Geometry check sheet. Reference: drawing and pictorial views, mm from the part's lowest x, y, z. A direction names the side the tool comes from. Give positions to 0.01 mm unless a question says otherwise; leave off trailing zeros. Write each loop counter-clockwise with the first axis right and the second up, starting at its lowest first coordinate (ties: lowest second). Pieces come first, ordered by that corner, then holes.
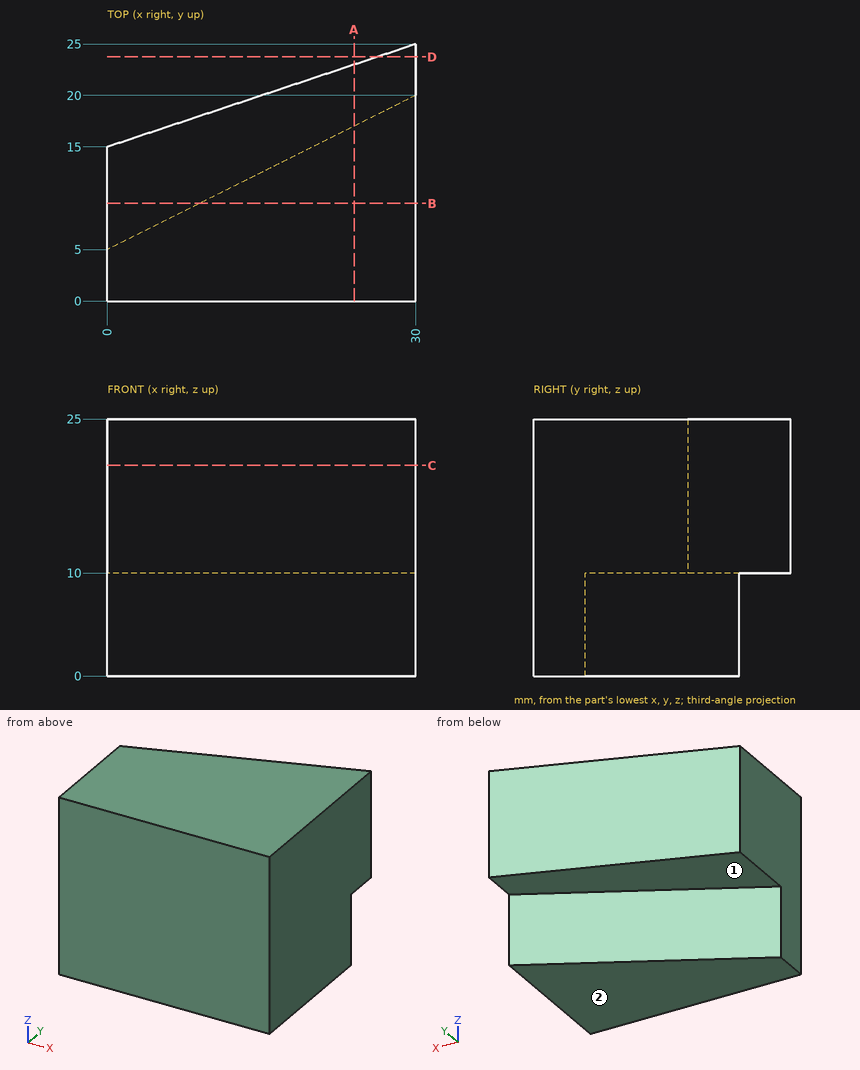
Item 1: Depth check by flat-ended pin: pin 1 (2 mm diameter, centred on y = 17.5, z = 8.5, fed in from -X); pin 2 (6 mm diameter, centred on x = 17, y = 17.5, fed in from -Z); pin 3 (1 mm diameter, centred on y = 15.5, z = 5.5, fed in from -X). Enter the tip coordinate at first touch or a pass-through.
Answer key:
pin 1: stops at x = 23
pin 2: stops at z = 10
pin 3: stops at x = 20
Item 2: Scan lines: line 1 along Z through (x, y) = (16.5, 16.25); line 2 along Y through (x, z) = (20, 5.5); line 3 along Y through (x, z) = (5, 16.25). Record each from-to range of solid material in increasing order.
Answer key:
line 1: z = 10 to 25
line 2: y = 0 to 15
line 3: y = 0 to 16.67
Item 3: Sectioned sample at B-B on y = 9.5. Record the cut outline in (x, z).
Answer key:
outline: (0, 10) - (9, 10) - (9, 0) - (30, 0) - (30, 25) - (0, 25) - close
Item 4: Sectioned sample at C-C on z = 20.5. Record the cut outline in (x, y).
Answer key:
outline: (0, 0) - (30, 0) - (30, 25) - (0, 15) - close
Item 5: Sectioned sample at D-D on y = 23.75. Record the cut outline in (x, z).
Answer key:
outline: (26.25, 10) - (30, 10) - (30, 25) - (26.25, 25) - close
Item 6: Sectioned sample at A-A on x = 24. Record the cut outline in (y, z).
Answer key:
outline: (0, 0) - (17, 0) - (17, 10) - (23, 10) - (23, 25) - (0, 25) - close
Item 7: Set-up check for the marked faces 1 and 2: record each of +Z, -Z, +X, -X, +Y, -Y from which the full face is reachable in a straight line by a thin tool's end or side.
Answer key:
face 1: -Z, -X, +Y
face 2: -Z, +X, -X, +Y, -Y
